Geometry check sheet. Reference: the model listing, model coordinates, mm. A direction names the side the tool comes from. Round coordinates to 2 decimals unless told otherwise and drop trailing zeros. Write each loop counter-clockwise with the first axis right and the second up, starting at its lowest first coordinate (ties: lowest second). Pieces come first, ordered by that corner, then holes. Notation, with made-up numbers: (-32.75, 11) -> (-8.75, 11) arc R29 cw to (-8.75, 46) -> close; hole circle Ø3 at (12.25, 88). An arc over 180 degrees is marked (long way). Return JSON: item names as keys, results as strings. Group by question number.
Autodesk Inventor part; units mm, degrees
ref_plane "YZ Plane" through (0, 0, 0) normal (1, 0, 0) x (0, 1, 0)
ref_plane "XZ Plane" through (0, 0, 0) normal (0, 1, 0) x (-1, 0, 0)
sketch "Sketch1" plane through (0, 0, 0) normal (1, 0, 0) x (0, 1, 0)
  circle A0 centre (0, 0) radius 23.114
  dimension "d0" = 46.228
extrude "Extrusion1" add sketch "Sketch1" along normal blind 5.588
sketch "Sketch3" plane through (0, 0, 0) normal (0, 0, 1) x (1, 0, 0)
  line L0 (5.588, -23.114) -> (5.588, 23.114)
  line L1 (5.588, 23.114) -> (5.588, 23.368)
  line L2 (5.588, 23.368) -> (5.334, 23.368)
  line L3 (5.334, 23.368) -> (5.334, 23.114)
  line L4 (0, 23.114) -> (5.588, 23.114)
  line L5 (5.334, 23.114) -> (5.588, 23.114)
  line L6 (0, 0) -> (5.588, 0)
  line L7 (0, 23.114) -> (0, 23.368)
  line L8 (0, 23.368) -> (0.254, 23.368)
  line L9 (0.254, 23.368) -> (0.254, 23.114)
  line L10 (0, 23.114) -> (0.254, 23.114)
  dimension "d5" = 0.254
  dimension "d6" = 0.254
  dimension "d7" = 0.254
  dimension "d8" = 0.254
revolve "Revolution1" add sketch "Sketch3" angle 360 about axis through (0, 0, 0) along (1, 0, 0)
sketch "Sketch4" plane through (5.588, 0, 0) normal (1, 0, 0) x (0, 0, -1)
  line L0 (0, -3.4925) -> (0, 3.4925) construction
  line L1 (2.413, -3.4925) -> (2.413, 3.4925)
  line L2 (-2.413, 3.4925) -> (-2.413, -3.4925)
  arc A0 (-2.413, -3.4925) -> (2.413, -3.4925) centre (0, -3.4925) ccw
  arc A1 (2.413, 3.4925) -> (-2.413, 3.4925) centre (0, 3.4925) ccw
  point P0 (0, 0)
  dimension "d10" = 3.4925
  dimension "d11" = 4.826
extrude "Extrusion2" cut sketch "Sketch4" against normal blind 5.08
properties part number "msheehan_wheel"
1) Tool access check on faces 1 (the face through (3.084, -5.905, 0.053)), 2 (the face through (0, 0, 0)). Record the directions out of +Z, -Z, +X, -X, +Y, -Y that give a thin tool (end or side, any length) a straight path to the whole face; none if there is none.
2) Sectioned sample at A-A on x = 1.3. Enter the section's corners in (y, z).
3) Material ranges on probe 1 along Z at (x, y) = (1.55, -5); probe 2 along Z at (x, y) = (0.3, 0); probe 3 along X at (y, z) = (2.5, -2), recorded low to high. Write a range as [from, to].
4) Sectioned sample at D-D on y = -9.5. Enter the section's corners in (x, z).
5) Sectioned sample at B-B on y = 0. Enter the section's corners in (x, z).
6) Go/stop test with flat-tipped pins: P1, Ø1.5, axis at x = 4, y = 0, coming from the +Z side; P2, Ø1.5, axis at x = 1.5, y = -8, coming from the -Z side; P3, Ø1.5, axis at x = 3, y = -0.5, coming from the -Z side. Record where each tip stops, or that it passes through.
7) Mould release check, pull along Y, two halves, no side actions. Record for faces 3 (the face through (2.758, 12.426, -19.49)), 4 (the face through (3, 0, 2.413)), 5 (the face through (5.588, 0, -5)): +Y half, -Y half, draft (parallel to the pull), parting line (faces both ways), or undercut.
8) Sectioned sample at C-C on z = -3. Enter the section's corners in (x, y).
Evaluation:
{
 "1": {"face 1": "+X", "face 2": "+Z, -Z, -X, +Y, -Y"},
 "2": {"outline": "circle Ø46.23 at (0, 0); hole (-3.49, -2.41) -> (3.49, -2.41) arc R2.41 ccw to (3.49, 2.41) -> (-3.49, 2.41) arc R2.41 ccw to start"},
 "3": {"probe 1": "z = [-22.57, -1.88], [1.88, 22.57]", "probe 2": "z = [-23.11, 23.11]", "probe 3": "x = [0, 0.51]"},
 "4": {"outline": "(0, -21.35) -> (0.25, -21.35) -> (0.25, -21.07) -> (5.33, -21.07) -> (5.33, -21.35) -> (5.59, -21.35) -> (5.59, 21.35) -> (5.33, 21.35) -> (5.33, 21.07) -> (0.25, 21.07) -> (0.25, 21.35) -> (0, 21.35) -> close"},
 "5": {"outline": "(0, -23.37) -> (0.25, -23.37) -> (0.25, -23.11) -> (5.33, -23.11) -> (5.33, -23.37) -> (5.59, -23.37) -> (5.59, -2.41) -> (0.51, -2.41) -> (0.51, 2.41) -> (5.59, 2.41) -> (5.59, 23.37) -> (5.33, 23.37) -> (5.33, 23.11) -> (0.25, 23.11) -> (0.25, 23.37) -> (0, 23.37) -> close"},
 "6": {"P1": "stops at z = 23.11", "P2": "stops at z = -21.95", "P3": "stops at z = -23.11"},
 "7": {"face 3": "parting line", "face 4": "undercut", "face 5": "draft"},
 "8": {"outline": "(0, -23.17) -> (0.25, -23.17) -> (0.25, -22.92) -> (5.33, -22.92) -> (5.33, -23.17) -> (5.59, -23.17) -> (5.59, 23.17) -> (5.33, 23.17) -> (5.33, 22.92) -> (0.25, 22.92) -> (0.25, 23.17) -> (0, 23.17) -> close"}
}
